Source: CAD feature listing. Evaluate the final solid. Frame: model axes, mm. A direction names the side the tool comes from. Coordinates: 2 decimals unless noted, no trailing zeros. Write each loop counter-clockwise with the first axis right and the second up, starting at its lowest first coordinate (ties: lowest second). Pieces come first, ordered by that corner, then holes. Notation, with made-up numbers: (73, -2) - (104, -2) arc R23 ccw to (104, 27) - close; hole circle Ø11 at (-32.75, -37). An arc over 180 degrees is marked (long way). One line per question, with ' | ' between items.
from build123d import *

# Parameters (mm, degrees)
F0_R        = 4.25
F0_W        = 8
F0_H        = 14.5
F0_W_2      = 3
F1_DEPTH    = 3
F2_DEPTH    = 12
F3_T1_DEPTH = 14.5
F3_T3_DEPTH = 29.5
F5_R        = 4.25
F6_DEPTH    = 22
F7_DEPTH    = 3
F8_T1_DEPTH = 28


# Not quite as in the source:
# - a fillet or chamfer that OpenCascade refuses, or shapes differently, is made with other operations: its cross-section is extruded or revolved along the edge and cut away or added


with BuildPart() as f1:
    # F0 (on Top) → F1 (new body)
    with BuildSketch(Plane.XY):
        with BuildLine():
            ThreePointArc((0, -7.25), (5.1265241636, -5.1265241636), (7.25, 0))
            ThreePointArc((7.25, 0), (5.1265241636, 5.1265241636), (0, 7.25))
            ThreePointArc((0, 7.25), (-7.25, 0), (0, -7.25))
        make_face()
        Circle(F0_R, mode=Mode.SUBTRACT)
        with BuildLine():
            Line((7.25, -7.25), (7.25, 0))
            ThreePointArc((7.25, 0), (5.1265241636, -5.1265241636), (0, -7.25))
            Line((0, -7.25), (7.25, -7.25))
        make_face()
        with BuildLine():
            ThreePointArc((0, 7.25), (5.1265241636, 5.1265241636), (7.25, 0))
            Line((7.25, 0), (7.25, 7.25))
            Line((7.25, 7.25), (0, 7.25))
        make_face()
        Polygon((7.25, 7.25), (7.25, 0), (7.25, -7.25), (7.35, -7.25), (7.35, 7.25), align=None)
        with Locations((11.35, 0)):
            Rectangle(F0_W, F0_H)
        with Locations((16.85, 0)):
            Rectangle(F0_W_2, F0_H)
    extrude(amount=F1_DEPTH)

    # F0 (on Top) → F2 (join)
    with BuildSketch(Plane.XY):
        with BuildLine():
            ThreePointArc((0, -7.25), (5.1265241636, -5.1265241636), (7.25, 0))
            ThreePointArc((7.25, 0), (5.1265241636, 5.1265241636), (0, 7.25))
            ThreePointArc((0, 7.25), (-7.25, 0), (0, -7.25))
        make_face()
        Circle(F0_R, mode=Mode.SUBTRACT)
        with BuildLine():
            ThreePointArc((0, 7.25), (5.1265241636, 5.1265241636), (7.25, 0))
            Line((7.25, 0), (7.25, 7.25))
            Line((7.25, 7.25), (0, 7.25))
        make_face()
        Polygon((7.25, 7.25), (7.25, 0), (7.25, -7.25), (7.35, -7.25), (7.35, 7.25), align=None)
        with Locations((16.85, 0)):
            Rectangle(F0_W_2, F0_H)
        with BuildLine():
            Line((7.25, -7.25), (7.25, 0))
            ThreePointArc((7.25, 0), (5.1265241636, -5.1265241636), (0, -7.25))
            Line((0, -7.25), (7.25, -7.25))
        make_face()
    extrude(amount=-F2_DEPTH)

    # F3: fillet of radius 3 on 3 edges, made by hand

    # F3_s2 → F3_t1 (join)
    with BuildSketch(Plane.XZ.offset(-7.25)):
        with BuildLine():
            ThreePointArc((7.35, -3), (8.2286796564, -0.8786796564), (10.35, 0))
            Line((10.35, 0), (7.35, 0))
            Line((7.35, 0), (7.35, -3))
        make_face()
        with BuildLine():
            ThreePointArc((12.35, 0), (14.4713203436, -0.8786796564), (15.35, -3))
            Line((15.35, -3), (15.35, 0))
            Line((15.35, 0), (12.35, 0))
        make_face()
    extrude(amount=F3_T1_DEPTH)

    # F3_s4 → F3_t3 (cut)
    with BuildSketch(Plane.XZ.offset(-14.75)):
        with BuildLine():
            ThreePointArc((15.35, 3), (17.4713203436, 2.1213203436), (18.35, 0))
            Line((18.35, 0), (18.35, 3))
            Line((18.35, 3), (15.35, 3))
        make_face()
    extrude(amount=F3_T3_DEPTH, mode=Mode.SUBTRACT)


with BuildPart() as f6:
    # F5 (on offset) → F6 (new body)
    with BuildSketch(Plane(origin=(0, 0, -37), x_dir=(1, 0, 0), z_dir=(0, 0, -1))):
        with BuildLine():
            Line((7.35, 7.25), (0, 7.25))
            ThreePointArc((0, 7.25), (-7.25, 0), (0, -7.25))
            Line((0, -7.25), (7.35, -7.25))
            Line((7.35, -7.25), (7.35, 7.25))
        make_face()
        Circle(F5_R, mode=Mode.SUBTRACT)
    extrude(amount=-F6_DEPTH)

    # F5 (on offset) → F7 (join)
    with BuildSketch(Plane(origin=(0, 0, -37), x_dir=(1, 0, 0), z_dir=(0, 0, -1))):
        with BuildLine():
            Line((7.35, 7.25), (0, 7.25))
            ThreePointArc((0, 7.25), (-7.25, 0), (0, -7.25))
            Line((0, -7.25), (7.35, -7.25))
            Line((7.35, -7.25), (7.35, 7.25))
        make_face()
        Circle(F5_R, mode=Mode.SUBTRACT)
        with BuildLine():
            ThreePointArc((0, -7.25), (-7.25, 0), (0, 7.25))
            Line((0, 7.25), (-37.25, 7.25))
            Line((-37.25, 7.25), (-37.25, 4))
            Line((-37.25, 4), (-22.25, 4))
            ThreePointArc((-22.25, 4), (-18.25, 0), (-22.25, -4))
            Line((-22.25, -4), (-37.25, -4))
            Line((-37.25, -4), (-37.25, -7.25))
            Line((-37.25, -7.25), (0, -7.25))
        make_face()
    extrude(amount=F7_DEPTH)

    # F8: fillet of radius 5 on 2 edges, made by hand

    # F8_s2 → F8_t1 (cut)
    with BuildSketch(Plane.XY.offset(-52.5)):
        with BuildLine():
            ThreePointArc((-32.25, -7.25), (-35.7855339059, -5.7855339059), (-37.25, -2.25))
            Line((-37.25, -2.25), (-37.25, -7.25))
            Line((-37.25, -7.25), (-32.25, -7.25))
        make_face()
        with BuildLine():
            ThreePointArc((-32.25, 7.25), (-35.7855339059, 5.7855339059), (-37.25, 2.25))
            Line((-37.25, 2.25), (-37.25, 7.25))
            Line((-37.25, 7.25), (-32.25, 7.25))
        make_face()
    extrude(amount=F8_T1_DEPTH, mode=Mode.SUBTRACT)


solid = f1.part
Item 1: Cut plane B-B on y = 0. Return loops of the section in (x, z).
Check sheet entries:
outline: (-7.25, -12) - (-4.25, -12) - (-4.25, 3) - (-7.25, 3) - close; (4.25, -12) - (7.35, -12) - (7.35, -3) arc R3 cw to (10.35, 0) - (12.35, 0) arc R3 cw to (15.35, -3) - (15.35, -12) - (18.35, -12) - (18.35, 0) arc R3 ccw to (15.35, 3) - (4.25, 3) - close
Item 2: Ray query, line 1 along X through (y, z) = (-1, -4.5); line 2 along X through (y, z) = (0.75, -1.5); line 3 along Y through (x, z) = (0, 1.55). Return the intervals inside material, ascending. Write a range as [from, to].
Check sheet entries:
line 1: [-7.18, -4.13], [4.13, 7.35], [15.35, 18.35] | line 2: [-7.21, -4.18], [4.18, 7.75], [14.95, 18.35] | line 3: [-7.25, -4.25], [4.25, 7.25]
Item 3: Mould query, pull axis X, two halves, no side actions, for faces 1 (the face through (17.45, 0.1, 2.14)), 2 (the face through (17, 0, -12)), 3 (the face through (14.45, 0.1, -0.86)), 4 (the face through (-7.25, 0.16, -4.39)). Classes: pulls with the +X half, pulls with the -X half, needs draft (parallel to the pull), parting line crosses it, or undercut.
Check sheet entries:
face 1: pulls with the +X half | face 2: needs draft | face 3: undercut | face 4: pulls with the -X half
Item 4: Pin query (flat end, axial travel): pin 1 Ø3 at (x, z) = (10.5, -2) entering from -Y; pin 2 Ø2 at (y, z) = (-3.5, -6) entering from -X; pin 3 Ø0.6 at (x, y) = (11, 1.5) entering from -Z; pin 4 Ø2 at (y, z) = (-5.5, -4) entering from -X. Return the tip coordinate at first contact, or that it passes through.
Check sheet entries:
pin 1: through | pin 2: x = -6.81 | pin 3: z = 0 | pin 4: x = -5.68
Item 5: Access query for faces 5 (the face through (6, 0, 3)), 6 (the face through (11, 0, 0)). Directions: +Z, -Z, +X, -X, +Y, -Y. A direction counts if a zero-diameter tool reaches every point of the face in a straight line with its end or side. Return the directions, or none.
Check sheet entries:
face 5: +Z, +X, -X, +Y, -Y | face 6: -Z, +Y, -Y
Item 6: Cut plane C-C on z = -1.25. Return loops of the section in (x, y), and give its area (3 significant figures).
Check sheet entries:
outline: (0, -7.25) - (7.91, -7.25) - (7.91, 7.25) - (0, 7.25) arc R7.25 ccw to start; (14.79, -7.25) - (18.35, -7.25) - (18.35, 7.25) - (14.79, 7.25) - close; hole circle Ø8.5 at (0, 0) | area: 192 mm²
Item 7: Cut plane A-A on z = -7. Return loops of the section in (x, y), and give its area (3 significant figures).
Check sheet entries:
outline: (0, -7.25) - (7.35, -7.25) - (7.35, 7.25) - (0, 7.25) arc R7.25 ccw to start; (15.35, -7.25) - (18.35, -7.25) - (18.35, 7.25) - (15.35, 7.25) - close; hole circle Ø8.5 at (0, 0) | area: 176 mm²
Item 8: Cut plane D-D on y = -2.5. Return loops of the section in (x, z), and give its area (3 significant figures).
Check sheet entries:
outline: (-6.81, -12) - (-3.44, -12) - (-3.44, 3) - (-6.81, 3) - close; (3.44, -12) - (7.35, -12) - (7.35, -3) arc R3 cw to (10.35, 0) - (12.35, 0) arc R3 cw to (15.35, -3) - (15.35, -12) - (18.35, -12) - (18.35, 0) arc R3 ccw to (15.35, 3) - (3.44, 3) - close | area: 180 mm²
